Here's how the part is built. I have some questions about the finished solid (model axes, mm). A direction names the side the tool comes from. Coordinates: 2 decimals unless noted, no trailing zeros. Loops run counter-clockwise (first coordinate to the right, second up) from the corner with the lowest first, then second, coordinate; pieces in that order, holes last. Notation, with made-up numbers: (-6, -10.75) -> (3, -10.75) arc R25 ccw to (3, 2.25) -> close; hole circle Ø11 at (4.5, 11.25). An arc over 180 degrees is marked (long way). Answer as a JSON object with one key per item and string values. Group by question number.
1) I want a section at D-D (z = 23). Write out the boundary of the cut face in (x, y) (3 decimals).
2) Which directions (+Z, -Z, +X, -X, +Y, -Y) give clear straight access to the entire face, cutting with the end or side of a thin tool? Please do faces 4 (the flat face through (-160.066, 11, 0)), 5 (the flat face through (-151, 13, 31.75)), 6 (the flat face through (-261, 5.556, -8)).
3) I want a section at C-C (x = -148.5). Write out the boundary of the cut face in (y, z) (3 decimals), then the cut area to 3 significant figures.
4) If we mould it in two halves opening along Z, with no side actions, what happens to faces 1 (the cylindrical face through (-236.4, 3.22, 38.34)), 2 (the flat face through (-151, 13, -31.75)), 3 (the flat face through (-208, 0, -1))? For each: +Z half, -Z half, draft (parallel to the pull), parting line (faces both ways), or undercut.
5) I'm going to push flat-ended pins straight in: pin 1 (5 mm diameter, centred on y = 10.5, z = 12, fed in from -X); pin 2 (1.5 mm diameter, centred on x = -168, y = 12, fed in from +Z); pin 3 (11 mm diameter, centred on x = -253.5, z = 1, fed in from +Y); pin 4 (11 mm diameter, centred on x = -231.75, z = -41.32, fed in from +Y). Where does each tip first touch, or does it pass through?
6) I want a section at A-A (z = 0). Write out the boundary of the cut face in (x, y) (3 decimals), then the cut area to 3 significant figures.
7) I want a section at B-B (y = 14.75). Write out the boundary of the cut face in (x, z).
8) I need wall thicknesses on probe 1 along Z at (x, y) = (-258.5, 9.5); probe 2 along Z at (x, y) = (-154.5, 9.75); probe 3 along X at (y, z) = (7.5, -4). Which ranges of each line are inside material? Lowest first, please. Write a range as [from, to].
```python
from build123d import *

# Parameters (mm, degrees)
SKETCH1_W               = 279.4
SKETCH1_H               = 101.6
BOSS_EXTRUDE1_DEPTH     = 6.35
SKETCH2_R               = 13.97
BOSS_EXTRUDE3_DEPTH     = 5.55625
SKETCH9_R               = 11.1125
CUT_EXTRUDE4_DEPTH      = 4.445
CUT_EXTRUDE5_START      = -5.55625
SKETCH10_R              = 11.1125
CUT_EXTRUDE5_DEPTH      = 5.55625
SKETCH11_R              = 7.9375
CUT_EXTRUDE6_DEPTH      = 285.078633923
SKETCH12_R              = 6.35
CUT_EXTRUDE7_DEPTH      = 285.051619429
SKETCH22_W              = 63.5
SKETCH22_H              = 63.5
BOSS_EXTRUDE7_DEPTH     = 12.7
SKETCH25_W              = 50.8
SKETCH25_H              = 50.8
CUT_EXTRUDE11_DEPTH     = 15.875
SKETCH32_R              = 4.7625
CUT_EXTRUDE12_DEPTH     = 6.35
SKETCH38_W              = 46.99
SKETCH38_H              = 18.470251096
CUT_EXTRUDE13_DEPTH     = 6.35
SKETCH60_R              = 4.7625
CUT_EXTRUDE23_DEPTH     = 6.35
CUT_EXTRUDE24_START     = -6.35
CUT_EXTRUDE24_OUTLINE_R = 4.7625
CUT_EXTRUDE24_DEPTH     = 19.05
SKETCH62_R              = 4.7625
CUT_EXTRUDE25_DEPTH     = 285.264471927


# Read off the part's stored shape, not the designer's step: Cut-Extrude24
with BuildPart() as part:
    # Sketch1 → Boss-Extrude1 (new body)
    with BuildSketch(Plane(origin=(0, 0, 0), x_dir=(1, 0, 0), z_dir=(0, 1, 0))):
        with Locations((-139.7, 0)):
            Rectangle(SKETCH1_W, SKETCH1_H)
    extrude(amount=BOSS_EXTRUDE1_DEPTH)

    # Sketch2 → Boss-Extrude3 (add)
    with BuildSketch(Plane(origin=(0, 6.35, 0), x_dir=(1, 0, 0), z_dir=(0, 1, 0))):
        with Locations(Location((-258.510557857, 0, 0), (0, 0, 90))):
            Circle(SKETCH2_R)
    extrude(amount=BOSS_EXTRUDE3_DEPTH)

    # Sketch9 → Cut-Extrude4 (cut)
    with BuildSketch(Plane(origin=(0, 11.90625, 0), x_dir=(1, 0, 0), z_dir=(0, 1, 0))):
        with Locations(Location((-258.510557857, 0, 0), (0, 0, 270))):
            Circle(SKETCH9_R)
    extrude(amount=-CUT_EXTRUDE4_DEPTH, mode=Mode.SUBTRACT)

    # Sketch10 → Cut-Extrude5 (cut)
    with BuildSketch(Plane(origin=(0, 0, 0), x_dir=(-1, 0, 0), z_dir=(0, -1, 0)).offset(CUT_EXTRUDE5_START)):
        with Locations(Location((258.510557857, 0, 0), (0, 0, 270))):
            Circle(SKETCH10_R)
    extrude(amount=CUT_EXTRUDE5_DEPTH, mode=Mode.SUBTRACT)

    # Sketch11 → Cut-Extrude6 (cut, through all)
    with BuildSketch(Plane(origin=(0, 7.46125, 0), x_dir=(1, 0, 0), z_dir=(0, 1, 0))):
        with Locations(Location((-258.510557857, 0, 0), (0, 0, 270))):
            Circle(SKETCH11_R)
    extrude(amount=-CUT_EXTRUDE6_DEPTH, mode=Mode.SUBTRACT)

    # Sketch12 → Cut-Extrude7 (cut, through all)
    with BuildSketch(Plane(origin=(0, 6.35, 0), x_dir=(1, 0, 0), z_dir=(0, 1, 0))):
        with Locations(Location((-134.666203771, 0, 0), (0, 0, 270))):
            Circle(SKETCH12_R)
    extrude(amount=-CUT_EXTRUDE7_DEPTH, mode=Mode.SUBTRACT)

    # Sketch22 → Boss-Extrude7 (add)
    with BuildSketch(Plane(origin=(0, 6.35, 0), x_dir=(1, 0, 0), z_dir=(0, 1, 0))):
        with Locations((-134.666203771, 0)):
            Rectangle(SKETCH22_W, SKETCH22_H)
    extrude(amount=BOSS_EXTRUDE7_DEPTH)

    # Sketch25 → Cut-Extrude11 (cut)
    with BuildSketch(Plane(origin=(0, 19.05, 0), x_dir=(1, 0, 0), z_dir=(0, 1, 0))):
        with Locations((-134.666203771, 0)):
            Rectangle(SKETCH25_W, SKETCH25_H)
    extrude(amount=-CUT_EXTRUDE11_DEPTH, mode=Mode.SUBTRACT)

    # Sketch32 → Cut-Extrude12 (cut)
    with BuildSketch(Plane(origin=(0, 6.35, 0), x_dir=(1, 0, 0), z_dir=(0, 1, 0))):
        with Locations(Location((-67.44195898, -40.64, 0), (0, 0, 270))):
            Circle(SKETCH32_R)
        with Locations(Location((-81.41195898, -40.64, 0), (0, 0, 270))):
            Circle(SKETCH32_R)
        with Locations(Location((-67.44195898, 40.64, 0), (0, 0, 270))):
            Circle(SKETCH32_R)
        with Locations(Location((-81.41195898, 40.64, 0), (0, 0, 270))):
            Circle(SKETCH32_R)
    extrude(amount=-CUT_EXTRUDE12_DEPTH, mode=Mode.SUBTRACT)

    # Sketch38 → Cut-Extrude13 (cut)
    with BuildSketch(Plane(origin=(0, 6.35, 0), x_dir=(1, 0, 0), z_dir=(0, 1, 0))):
        with Locations((-23.495, -24.777709652)):
            Rectangle(SKETCH38_W, SKETCH38_H)
    extrude(amount=-CUT_EXTRUDE13_DEPTH, mode=Mode.SUBTRACT)

    # Sketch60 → Cut-Extrude23 (cut)
    with BuildSketch(Plane(origin=(0, 6.35, 0), x_dir=(1, 0, 0), z_dir=(0, 1, 0))):
        with Locations(Location((-231.7492444, 41.324145444, 0), (0, 0, 270))):
            Circle(SKETCH60_R)
        with Locations(Location((-231.7492444, -39.369341378, 0), (0, 0, 270))):
            Circle(SKETCH60_R)
        with Locations(Location((-173.509244294, -39.369341378, 0), (0, 0, 270))):
            Circle(SKETCH60_R)
        with Locations(Location((-173.509244294, 41.324145444, 0), (0, 0, 270))):
            Circle(SKETCH60_R)
    extrude(amount=-CUT_EXTRUDE23_DEPTH, mode=Mode.SUBTRACT)

    # Cut-Extrude24 outline → Cut-Extrude24 (cut)
    with BuildSketch(Plane(origin=(0, 6.35, 0), x_dir=(1, 0, 0), z_dir=(0, 1, 0)).offset(CUT_EXTRUDE24_START)):
        with BuildLine():
            Line((-134.666203771, -50.8), (0, -50.8))
            Line((0, -50.8), (0, -34.0128352))
            Line((0, -34.0128352), (-46.99, -34.0128352))
            Line((-46.99, -34.0128352), (-46.99, -15.542584104))
            Line((-46.99, -15.542584104), (0, -15.542584104))
            Line((0, -15.542584104), (0, 50.8))
            Line((0, 50.8), (-134.666203771, 50.8))
            Line((-134.666203771, 50.8), (-134.666203771, 6.35))
            ThreePointArc((-134.666203771, 6.35), (-128.316203771, 0), (-134.666203771, -6.35))
            Line((-134.666203771, -6.35), (-134.666203771, -50.8))
        make_face()
        with Locations((-81.41195898, -40.64)):
            Circle(CUT_EXTRUDE24_OUTLINE_R, mode=Mode.SUBTRACT)
        with Locations((-67.44195898, -40.64)):
            Circle(CUT_EXTRUDE24_OUTLINE_R, mode=Mode.SUBTRACT)
        with Locations((-81.41195898, 40.64)):
            Circle(CUT_EXTRUDE24_OUTLINE_R, mode=Mode.SUBTRACT)
        with Locations((-67.44195898, 40.64)):
            Circle(CUT_EXTRUDE24_OUTLINE_R, mode=Mode.SUBTRACT)
    extrude(amount=CUT_EXTRUDE24_DEPTH, mode=Mode.SUBTRACT)

    # Sketch62 → Cut-Extrude25 (cut, through all)
    with BuildSketch(Plane(origin=(0, 6.35, 0), x_dir=(1, 0, 0), z_dir=(0, 1, 0))):
        with Locations(Location((-145.334203771, 41.275, 0), (0, 0, 270))):
            Circle(SKETCH62_R)
    cut_extrude25 = extrude(amount=-CUT_EXTRUDE25_DEPTH, mode=Mode.SUBTRACT)

    # Mirror1: Cut-Extrude25 across plane
    add(cut_extrude25.mirror(Plane.XY), mode=Mode.SUBTRACT)


solid = part.part
```
Determined:
{
 "1": {"outline": "(-279.4, 0) -> (-134.666, 0) -> (-134.666, 3.175) -> (-160.066, 3.175) -> (-160.066, 19.05) -> (-166.416, 19.05) -> (-166.416, 6.35) -> (-279.4, 6.35) -> close"},
 "2": {"face 4": "+X, +Y", "face 5": "+Z, +X, -X, +Y", "face 6": "-Y"},
 "3": {"outline": "(0, -50.8) -> (6.35, -50.8) -> (6.35, -44.833) -> (0, -44.833) -> close; (0, -37.717) -> (6.35, -37.717) -> (6.35, -31.75) -> (19.05, -31.75) -> (19.05, -25.4) -> (3.175, -25.4) -> (3.175, 25.4) -> (19.05, 25.4) -> (19.05, 31.75) -> (6.35, 31.75) -> (6.35, 37.717) -> (0, 37.717) -> close; (0, 44.833) -> (6.35, 44.833) -> (6.35, 50.8) -> (0, 50.8) -> close", "area": "555 mm^2"},
 "4": {"face 1": "undercut", "face 2": "-Z half", "face 3": "draft"},
 "5": {"pin 1": "x = -268.75", "pin 2": "through", "pin 3": "y = 7.46", "pin 4": "y = 6.35"},
 "6": {"outline": "(-279.4, 0) -> (-269.623, 0) -> (-269.623, 5.556) -> (-266.448, 5.556) -> (-266.448, 7.461) -> (-269.623, 7.461) -> (-269.623, 11.906) -> (-272.481, 11.906) -> (-272.481, 6.35) -> (-279.4, 6.35) -> close; (-250.573, 5.556) -> (-247.398, 5.556) -> (-247.398, 0) -> (-141.016, 0) -> (-141.016, 3.175) -> (-160.066, 3.175) -> (-160.066, 19.05) -> (-166.416, 19.05) -> (-166.416, 6.35) -> (-244.541, 6.35) -> (-244.541, 11.906) -> (-247.398, 11.906) -> (-247.398, 7.461) -> (-250.573, 7.461) -> close", "area": "802 mm^2"},
 "7": {"outline": "(-166.42, -31.75) -> (-134.67, -31.75) -> (-134.67, -25.4) -> (-160.07, -25.4) -> (-160.07, 25.4) -> (-134.67, 25.4) -> (-134.67, 31.75) -> (-166.42, 31.75) -> close"},
 "8": {"probe 1": "[-13.97, -11.11], [11.11, 13.97]", "probe 2": "[-31.75, -25.4], [25.4, 31.75]", "probe 3": "[-271.9, -268.88], [-248.14, -245.13], [-166.42, -160.07]"}
}
